```python
from build123d import *

# Parameters (mm, degrees)
SKETCH1_W            = 40
SKETCH1_H            = 40
SKETCH1_R            = 0.9
BOSS_EXTRUDE1_DEPTH  = 6
SKETCH11_W           = 40
SKETCH11_H           = 40
SKETCH11_R           = 5
BOSS_EXTRUDE6_DEPTH  = 7
SKETCH13_R           = 1.5
SKETCH13_R_2         = 1.395390764
CUT_EXTRUDE5_DEPTH   = 27
SKETCH13_3_R         = 3
SKETCH13_3_R_2       = 1.5
CUT_EXTRUDE6_DEPTH   = 3
SKETCH15_R           = 2.5
CUT_EXTRUDE9_DEPTH   = 5
CIRPATTERN4_COUNT    = 4
SKETCH16_R           = 3
BOSS_EXTRUDE7_DEPTH  = 13
SKETCH17_R           = 2.5
BOSS_EXTRUDE8_DEPTH  = 5
SKETCH18_R           = 2.5
BOSS_EXTRUDE9_DEPTH  = 5
SKETCH19_R           = 2.5
BOSS_EXTRUDE10_DEPTH = 5
SKETCH20_R           = 2.5
BOSS_EXTRUDE11_DEPTH = 5
SKETCH21_R           = 1.5
CUT_EXTRUDE10_DEPTH  = 25
SKETCH21_3_R         = 2.5
SKETCH21_3_R_2       = 1.5
CUT_EXTRUDE11_DEPTH  = 5
SKETCH22_R           = 1
CUT_EXTRUDE12_DEPTH  = 7
CIRPATTERN5_COUNT    = 4


with BuildPart() as part:
    # Sketch1 → Boss-Extrude1 (new body)
    with BuildSketch(Plane(origin=(0, 0, 0), x_dir=(0, 1, 0), z_dir=(0, 0, 1))):
        Rectangle(SKETCH1_W, SKETCH1_H)
        with Locations(Location((10.5, 0, 0), (0, 0, 270))):
            Circle(SKETCH1_R, mode=Mode.SUBTRACT)
        with Locations(Location((-10.5, 12.5, 0), (0, 0, 270))):
            Circle(SKETCH1_R, mode=Mode.SUBTRACT)
        with Locations(Location((-10.5, 0, 0), (0, 0, 270))):
            Circle(SKETCH1_R, mode=Mode.SUBTRACT)
        with Locations(Location((10.5, 12.5, 0), (0, 0, 270))):
            Circle(SKETCH1_R, mode=Mode.SUBTRACT)
        Polygon((-5, -13), (-8, -13), (-8, -5), (-5, -5), (-5, 5), (5, 5), (5, -5), (5, -13), align=None, mode=Mode.SUBTRACT)
    extrude(amount=BOSS_EXTRUDE1_DEPTH)

    # Sketch11 → Boss-Extrude6 (add)
    with BuildSketch(Plane.XY.offset(6)):
        Rectangle(SKETCH11_W, SKETCH11_H)
        with Locations(Location((0, 0, 0), (0, 0, 180))):
            Circle(SKETCH11_R, mode=Mode.SUBTRACT)
    extrude(amount=BOSS_EXTRUDE6_DEPTH)

    # Sketch13 → Cut-Extrude5 (cut)
    with BuildSketch(Plane(origin=(0, 0, 0), x_dir=(1, 0, 0), z_dir=(0, 0, -1))):
        with Locations(Location((-6.25, 13.75, 0), (0, 0, 180))):
            Circle(SKETCH13_R)
        with Locations(Location((6.25, 13.75, 0), (0, 0, 180))):
            Circle(SKETCH13_R)
        with Locations(Location((6.25, -13.75, 0), (0, 0, 180))):
            Circle(SKETCH13_R_2)
        with Locations(Location((-6.25, -13.75, 0), (0, 0, 180))):
            Circle(SKETCH13_R)
    extrude(amount=-CUT_EXTRUDE5_DEPTH, mode=Mode.SUBTRACT)

    # Sketch13<3> → Cut-Extrude6 (cut)
    # profile 1 of 4: a face of its own
    with BuildSketch(Plane(origin=(0, 0, 0), x_dir=(1, 0, 0), z_dir=(0, 0, -1))):
        with Locations(Location((-6.25, -13.75, 0), (0, 0, 180))):
            Circle(SKETCH13_3_R)
        with Locations(Location((-6.25, -13.75, 0), (0, 0, 180))):
            Circle(SKETCH13_3_R_2, mode=Mode.SUBTRACT)
    # profile 2 of 4: a face of its own
    with BuildSketch(Plane(origin=(0, 0, 0), x_dir=(1, 0, 0), z_dir=(0, 0, -1))):
        with Locations(Location((6.25, 13.75, 0), (0, 0, 180))):
            Circle(SKETCH13_3_R)
        with Locations(Location((6.25, 13.75, 0), (0, 0, 180))):
            Circle(SKETCH13_3_R_2, mode=Mode.SUBTRACT)
    # profile 3 of 4: a face of its own
    with BuildSketch(Plane(origin=(0, 0, 0), x_dir=(1, 0, 0), z_dir=(0, 0, -1))):
        with Locations(Location((-6.25, 13.75, 0), (0, 0, 180))):
            Circle(SKETCH13_3_R)
        with Locations(Location((-6.25, 13.75, 0), (0, 0, 180))):
            Circle(SKETCH13_3_R_2, mode=Mode.SUBTRACT)
    # profile 4 of 4: a face of its own
    with BuildSketch(Plane(origin=(0, 0, 0), x_dir=(1, 0, 0), z_dir=(0, 0, -1))):
        with Locations(Location((6.25, -13.75, 0), (0, 0, 180))):
            Circle(SKETCH13_3_R)
    extrude(amount=-CUT_EXTRUDE6_DEPTH, mode=Mode.SUBTRACT)

    # Sketch15 → Cut-Extrude9 (cut)
    with BuildSketch(Plane(origin=(0, 20, 0), x_dir=(-1, 0, 0), z_dir=(0, 1, 0))):
        with Locations(Location((-13.5, 6.5, 0), (0, 0, 90))):
            Circle(SKETCH15_R)
        with Locations(Location((13.5, 6.5, 0), (0, 0, 270))):
            Circle(SKETCH15_R)
    cut_extrude9 = extrude(amount=-CUT_EXTRUDE9_DEPTH, mode=Mode.SUBTRACT)

    # CirPattern4: Cut-Extrude9 ×4 about axis
    cirpattern4_axis = Axis((0, 0, 0), (0, 0, 1))
    for i in range(1, CIRPATTERN4_COUNT):
        add(cut_extrude9.rotate(cirpattern4_axis, i * 360 / CIRPATTERN4_COUNT), mode=Mode.SUBTRACT)

    # Sketch16 → Boss-Extrude7 (add)
    with BuildSketch(Plane(origin=(0, 0, 0), x_dir=(1, 0, 0), z_dir=(0, 0, -1))):
        with Locations((-6.25, 13.75)):
            Circle(SKETCH16_R)
        with Locations((6.25, 13.75)):
            Circle(SKETCH16_R)
        with Locations((-6.25, -13.75)):
            Circle(SKETCH16_R)
        with Locations((6.25, -13.75)):
            Circle(SKETCH16_R)
    extrude(amount=-BOSS_EXTRUDE7_DEPTH)

    # Sketch17 → Boss-Extrude8 (add)
    with BuildSketch(Plane(origin=(0, 20, 0), x_dir=(-1, 0, 0), z_dir=(0, 1, 0))):
        with Locations(Location((-13.5, 6.5, 0), (0, 0, 270))):
            Circle(SKETCH17_R)
        with Locations(Location((13.5, 6.5, 0), (0, 0, 306.869897646))):
            Circle(SKETCH17_R)
    extrude(amount=-BOSS_EXTRUDE8_DEPTH)

    # Sketch18 → Boss-Extrude9 (add)
    with BuildSketch(Plane(origin=(-20, 0, 0), x_dir=(0, -1, 0), z_dir=(-1, 0, 0))):
        with Locations(Location((-13.5, 6.5, 0), (0, 0, 233.130102354))):
            Circle(SKETCH18_R)
        with Locations(Location((13.5, 6.5, 0), (0, 0, 90))):
            Circle(SKETCH18_R)
    extrude(amount=-BOSS_EXTRUDE9_DEPTH)

    # Sketch19 → Boss-Extrude10 (add)
    with BuildSketch(Plane.XZ.offset(20)):
        with Locations((-13.5, 6.5)):
            Circle(SKETCH19_R)
        with Locations((13.5, 6.5)):
            Circle(SKETCH19_R)
    extrude(amount=-BOSS_EXTRUDE10_DEPTH)

    # Sketch20 → Boss-Extrude11 (add)
    with BuildSketch(Plane.YZ.offset(20)):
        with Locations((-13.5, 6.5)):
            Circle(SKETCH20_R)
        with Locations((13.5, 6.5)):
            Circle(SKETCH20_R)
    extrude(amount=-BOSS_EXTRUDE11_DEPTH)

    # Sketch21 → Cut-Extrude10 (cut)
    with BuildSketch(Plane(origin=(0, 0, 0), x_dir=(1, 0, 0), z_dir=(0, 0, -1))):
        with Locations(Location((-5, 15, 0), (0, 0, 180))):
            Circle(SKETCH21_R)
        with Locations(Location((15, 15, 0), (0, 0, 180))):
            Circle(SKETCH21_R)
        with Locations(Location((15, -15, 0), (0, 0, 180))):
            Circle(SKETCH21_R)
        with Locations(Location((-5, -15, 0), (0, 0, 180))):
            Circle(SKETCH21_R)
    extrude(amount=-CUT_EXTRUDE10_DEPTH, mode=Mode.SUBTRACT)

    # Sketch21<3> → Cut-Extrude11 (cut)
    # profile 1 of 4: a face of its own
    with BuildSketch(Plane(origin=(0, 0, 0), x_dir=(1, 0, 0), z_dir=(0, 0, -1))):
        with Locations(Location((-5, 15, 0), (0, 0, 180))):
            Circle(SKETCH21_3_R)
        with Locations(Location((-5, 15, 0), (0, 0, 180))):
            Circle(SKETCH21_3_R_2, mode=Mode.SUBTRACT)
    # profile 2 of 4: a face of its own
    with BuildSketch(Plane(origin=(0, 0, 0), x_dir=(1, 0, 0), z_dir=(0, 0, -1))):
        with Locations(Location((15, 15, 0), (0, 0, 180))):
            Circle(SKETCH21_3_R)
        with Locations(Location((15, 15, 0), (0, 0, 180))):
            Circle(SKETCH21_3_R_2, mode=Mode.SUBTRACT)
    # profile 3 of 4: a face of its own
    with BuildSketch(Plane(origin=(0, 0, 0), x_dir=(1, 0, 0), z_dir=(0, 0, -1))):
        with Locations(Location((15, -15, 0), (0, 0, 180))):
            Circle(SKETCH21_3_R)
        with Locations(Location((15, -15, 0), (0, 0, 180))):
            Circle(SKETCH21_3_R_2, mode=Mode.SUBTRACT)
    # profile 4 of 4: a face of its own
    with BuildSketch(Plane(origin=(0, 0, 0), x_dir=(1, 0, 0), z_dir=(0, 0, -1))):
        with Locations(Location((-5, -15, 0), (0, 0, 180))):
            Circle(SKETCH21_3_R)
        with Locations(Location((-5, -15, 0), (0, 0, 180))):
            Circle(SKETCH21_3_R_2, mode=Mode.SUBTRACT)
    extrude(amount=-CUT_EXTRUDE11_DEPTH, mode=Mode.SUBTRACT)

    # Sketch22 → Cut-Extrude12 (cut)
    with BuildSketch(Plane(origin=(0, 20, 0), x_dir=(-1, 0, 0), z_dir=(0, 1, 0))):
        with Locations(Location((-10, 6.5, 0), (0, 0, 90))):
            Circle(SKETCH22_R)
        with Locations(Location((10, 6.5, 0), (0, 0, 270))):
            Circle(SKETCH22_R)
    cut_extrude12 = extrude(amount=-CUT_EXTRUDE12_DEPTH, mode=Mode.SUBTRACT)

    # CirPattern5: Cut-Extrude12 ×4 about axis
    cirpattern5_axis = Axis((0, 0, 0), (0, 0, 1))
    for i in range(1, CIRPATTERN5_COUNT):
        add(cut_extrude12.rotate(cirpattern5_axis, i * 360 / CIRPATTERN5_COUNT), mode=Mode.SUBTRACT)


solid = part.part
```
Could you check a few things on this model? Use its own coordinates, in mm. A direction names the side the tool comes from. Round coordinates to 2 decimals unless told otherwise and drop trailing zeros. Loops run counter-clockwise (first coordinate to the right, second up) from the corner with the lowest first, then second, coordinate; pieces in that order, holes last.
Q1. For P1, Ø1.6, axis at x = 10, z = 6.5, coming from the -Y side; P2, Ø3, axis at y = 10, z = 6.5, coming from the +X side; P3, Ø1.8, axis at x = 15, y = 15, coming from the -Z side; P4, Ø0.5, axis at x = -12.5, y = -10.5, coming from the -Z side, each with a flat end and sliding along its axis, tell me the tip position at first contact or that it passes through.
Q2. I want a section at B-B (y = 4). Write out the boundary of the cut face in (x, z), and give its area (3 significant figures).
Q3. Thinking about a two-plate mould opening in Z: for faces 1 (the cylindrical face through (-6.386, -15.575, 8.944)), 2 (the flat face through (0, -10, 6)), 3 (the flat face through (13, 10, 7)), which applies, pulls with the +Z half, pulls with the -Z half, needs draft (parallel to the pull), parting line crosses it, or undercut?
Q4. On a 3-axis mill with a long thin cutter (end or side, diameter ignored), from which of +Z, -Z, +X, -X, +Y, -Y can I reach the whole of each face in a straight line? I mean faces 4 (the flat face through (10, 13, 6)), 5 (the cylindrical face through (-16.55, 10.99, 6.37)), 6 (the cylindrical face through (-10.99, -16.55, 6.37)), 7 (the cylindrical face through (17, 13.5, 2.5)), 8 (the cylindrical face through (16.5, -9.4, 5.7)). Say none if no direction works.
Q5. Please list where these lines run through material, in increasing order: L1, parallel to X at y = -6.5, z = 1; L2, parallel to Y at x = 0, z = 4.5; L3, parallel to Y at x = 0, z = 9.
Q6. I want a section at D-D (x = 10.5). Write out the boundary of the cut face in (y, z).
Q7. I want a section at C-C (z = 8). Write out the boundary of the cut face in (x, y), and give its area (3 significant figures).
Q8. I want a section at A-A (x = 15). Write out the boundary of the cut face in (y, z).
Answer below:
1. P1: stops at y = -13
1. P2: stops at x = 20
1. P3: passes through
1. P4: stops at z = 6
2. outline: (-20, 0) - (-5, 0) - (-5, 6) - (-3, 6) - (-3, 13) - (-20, 13) - close; (3, 6) - (13, 6) - (13, 0) - (20, 0) - (20, 13) - (3, 13) - close
2. area: 370 mm2
3. face 1: needs draft
3. face 2: pulls with the -Z half
3. face 3: undercut
4. face 4: +Y
4. face 5: -X
4. face 6: -Y
4. face 7: -Z
4. face 8: +X
5. L1: x = -20 to 5, 13 to 20
5. L2: y = -20 to -11.4, -9.6 to -5, 5 to 9.6, 11.4 to 20
5. L3: y = -20 to -5, 5 to 20
6. outline: (-20, 0) - (-8, 0) - (-8, 6) - (5, 6) - (5, 0) - (20, 0) - (20, 5.63) - (13, 5.63) - (13, 7.37) - (20, 7.37) - (20, 13) - (-20, 13) - (-20, 7.37) - (-13, 7.37) - (-13, 5.63) - (-20, 5.63) - close
7. outline: (-20, -20) - (20, -20) - (20, 20) - (-20, 20) - close; hole circle Ø3 at (-5, -15); hole circle Ø3 at (-5, 15); hole circle Ø10 at (0, 0); hole circle Ø3 at (15, -15); hole circle Ø3 at (15, 15)
7. area: 1,490 mm2
8. outline: (-20, 0) - (-17.5, 0) - (-17.5, 5) - (-16.5, 5) - (-16.5, 13) - (-20, 13) - close; (-13.5, 5) - (-12.5, 5) - (-12.5, 0) - (12.5, 0) - (12.5, 5) - (13.5, 5) - (13.5, 13) - (-13.5, 13) - close; (16.5, 5) - (17.5, 5) - (17.5, 0) - (20, 0) - (20, 13) - (16.5, 13) - close; hole circle Ø2 at (-10, 6.5); hole circle Ø2 at (10, 6.5)
